from build123d import *

# Parameters (mm, degrees)
F0_W     = 1
F0_H     = 8
F0_H_2   = 12
F0_W_2   = 18
F1_DEPTH = 0.9
F2_DEPTH = 12
F3_R     = 2
F5_DEPTH = 1
F7_DEPTH = 1
F8_W     = 1.2
F8_H     = 4
F9_DEPTH = 25


with BuildPart() as f1:
    # F0 (on Top) → F1 (new body)
    with BuildSketch(Plane.XY):
        with BuildLine():
            Line((-10, 14), (-20.5, 14))
            ThreePointArc((-20.5, 14), (-24.0355339059, 12.5355339059), (-25.5, 9))
            Line((-25.5, 9), (-25.5, 6))
            Line((-25.5, 6), (-10, 6))
            Line((-10, 6), (-10, 14))
        make_face()
        with Locations((-9.5, 10)):
            Rectangle(F0_W, F0_H)
        with Locations((-9.5, 0)):
            Rectangle(F0_W, F0_H_2)
        with Locations((-9.5, -10)):
            Rectangle(F0_W, F0_H)
        with BuildLine():
            Line((-10, -14), (-10, -6))
            Line((-10, -6), (-25.5, -6))
            Line((-25.5, -6), (-25.5, -9))
            ThreePointArc((-25.5, -9), (-24.0355339059, -12.5355339059), (-20.5, -14))
            Line((-20.5, -14), (-10, -14))
        make_face()
        with BuildLine():
            Line((25.5, -6), (10, -6))
            Line((10, -6), (10, -14))
            Line((10, -14), (20.5, -14))
            ThreePointArc((20.5, -14), (24.0355339059, -12.5355339059), (25.5, -9))
            Line((25.5, -9), (25.5, -6))
        make_face()
        with BuildLine():
            Line((20.5, 14), (10, 14))
            Line((10, 14), (10, 6))
            Line((10, 6), (25.5, 6))
            Line((25.5, 6), (25.5, 9))
            ThreePointArc((25.5, 9), (24.0355339059, 12.5355339059), (20.5, 14))
        make_face()
        with Locations((9.5, 10)):
            Rectangle(F0_W, F0_H)
        with Locations((9.5, 0)):
            Rectangle(F0_W, F0_H_2)
        with Locations((9.5, -10)):
            Rectangle(F0_W, F0_H)
        Rectangle(F0_W_2, F0_H_2)
    extrude(amount=F1_DEPTH)

    # F0 (on Top) → F2 (join)
    with BuildSketch(Plane.XY):
        with Locations((-9.5, -10)):
            Rectangle(F0_W, F0_H)
        with Locations((-9.5, 0)):
            Rectangle(F0_W, F0_H_2)
        with Locations((-9.5, 10)):
            Rectangle(F0_W, F0_H)
        with Locations((9.5, 10)):
            Rectangle(F0_W, F0_H)
        with Locations((9.5, 0)):
            Rectangle(F0_W, F0_H_2)
        with Locations((9.5, -10)):
            Rectangle(F0_W, F0_H)
    extrude(amount=F2_DEPTH)

    # F3
    f3_edges = [f1.edges().sort_by_distance(p)[0] for p in [
        (-25.5, 6, 0.45),
        (-10, 6, 0.45),
        (-10, -6, 0.45),
        (-25.5, -6, 0.45),
        (-9, 6, 0.45),
        (9, 6, 0.45),
        (25.5, 6, 0.45),
        (25.5, -6, 0.45),
        (10, 6, 0.45),
        (10, -6, 0.45),
        (9, -6, 0.45),
        (-9, -6, 0.45),
    ]]
    fillet(f3_edges, radius=F3_R)

    # F4 (on face) → F5 (join)
    with BuildSketch(Plane.YZ.offset(10)):
        Polygon((-14.9711241651, 12), (-14, 0.9), (-14, 12), align=None)
        Polygon((14.9711241651, 12), (14, 12), (14, 0.9), align=None)
    extrude(amount=-F5_DEPTH)

    # F6 (on face) → F7 (join)
    with BuildSketch(Plane(origin=(-10, 0, 0), x_dir=(0, -1, 0), z_dir=(-1, 0, 0))):
        Polygon((-14, 0.9), (-14, 12), (-14.9711241651, 12), align=None)
        Polygon((14.9711241651, 12), (14, 12), (14, 0.9), align=None)
    extrude(amount=-F7_DEPTH)

    # F8 (on face) → F9 (cut)
    with BuildSketch(Plane.YZ.offset(10)):
        with Locations((0, 10)):
            Rectangle(F8_W, F8_H)
    extrude(amount=-F9_DEPTH, mode=Mode.SUBTRACT)


solid = f1.part
Verification items for the finished model (mm, model axes). A direction names the side the tool comes from. Give positions to 0.01 mm unless a question says otherwise; leave off trailing zeros. Write each loop counter-clockwise with the first axis right and the second up, starting at its lowest first coordinate (ties: lowest second). Pieces come first, ordered by that corner, then holes.
(1) Cross-section at A-A (y = 8.5). Enter the section's corners in (x, z).
(2) Access from +Z, -Z, +X, -X, +Y, -Y to the whole of each face (thin tool, end or side, straight path). Record for faces 4 (the face through (24.9, 6.57, 0.46)), 5 (the face through (8.43, 6.6, 0.46)), 6 (the face through (0, 0, 0.9)), 7 (the face through (-9.5, 0, 8)).
(3) Gauge pin test, flat ends, axial feed: pin 1 (1.1 mm diameter, centred on x = 9.5, z = 9.5, fed in from -Y); pin 2 (1.5 mm diameter, centred on y = 1.5, z = 2, fed in from -X); pin 3 (0.7 mm diameter, centred on x = 15.5, z = 0.5, fed in from -Y). Record the tip position at first contact, or that the pin passes through.
(4) Cross-section at B-B (z = 4). Enter the section's corners in (x, y).
(5) Cross-section at D-D (y = -2). Enter the section's corners in (x, z), plus the area to 3 significant figures.
(6) Material ranges on line 1 (X direction, y = 8.25, z = 1.5); line 2 (Z direction, x = 14, y = 9.75), recorded low to high.
(7) Mould release check, pull along Y, two halves, no side actions. Record for faces 1 (the face through (9.51, 14.48, 6.37)), 2 (the face through (-18, -10, 0.9)), 3 (the face through (-24.93, 6.6, 0.46)): +Y half, -Y half, draft (parallel to the pull), parting line (faces both ways), or undercut.
(8) Cross-section at C-C (x = -15). Enter the section's corners in (y, z), plus the area to 3 significant figures.
Worked out:
1. outline: (-25.5, 0) - (-9, 0) - (-9, 12) - (-10, 12) - (-10, 0.9) - (-25.5, 0.9) - close; (9, 0) - (25.5, 0) - (25.5, 0.9) - (10, 0.9) - (10, 12) - (9, 12) - close
2. face 4: +Z, -Z, +X
2. face 5: +Z, -Z, +Y
2. face 6: +Z, +Y, -Y
2. face 7: +Z, +X, -X
3. pin 1: stops at y = -14.8
3. pin 2: stops at x = -10
3. pin 3: stops at y = -14
4. outline: (-10, -14.27) - (-9, -14.27) - (-9, 14.27) - (-10, 14.27) - close; (9, -14.27) - (10, -14.27) - (10, 14.27) - (9, 14.27) - close
5. outline: (-10, 0) - (10, 0) - (10, 12) - (9, 12) - (9, 0.9) - (-9, 0.9) - (-9, 12) - (-10, 12) - close
5. area: 40.2 mm2
6. line 1: x = -10 to -9, 9 to 10
6. line 2: z = 0 to 0.9
7. face 1: +Y half
7. face 2: draft
7. face 3: undercut
8. outline: (-14, 0) - (-6, 0) - (-6, 0.9) - (-14, 0.9) - close; (6, 0) - (14, 0) - (14, 0.9) - (6, 0.9) - close
8. area: 14.4 mm2
